The listing builds one solid part. Answer for the finished solid, in the listing's coordinates (mm). Face numbers are marked on the shaded views. A direction names the side the tool comes from. Coordinates: 2 decimals unless noted, no trailing zeros. Order: outer loops, then holes, each group sorted by start corner. A loop starts at its lowest first (then second) coordinate and runs counter-clockwise, first axis right, second up. Notation, with made-up numbers: (2.5, 16) -> (14.5, 16) arc R21 cw to (14.5, 27) -> close; hole circle Ø1 at (14.25, -11). An arc over 180 degrees is marked (long way). Answer in a Markdown table with one row per item.
Autodesk Fusion 360 part; units mm, degrees
sketch "Sketch1" plane through (0, 0, 0) normal (1, 0, 0) x (0, 1, 0)
  line L0 (0, 0) -> (-30, 0)
  line L1 (-30, 0) -> (-30, 15.5)
  line L2 (-30, 15.5) -> (0, 15.5)
  line L3 (0, 15.5) -> (0, 0)
  circle A0 centre (-4, 10.5) radius 1.6
  circle A1 centre (-24, 10.5) radius 1.6
  dimension "d1" = 30
  dimension "d2" = 15.5
  dimension "d3" = 3.2
  dimension "d4" = 3.2
  dimension "d5" = 20
  dimension "d6" = 4
  dimension "d7" = 5
extrude "Extrude1" add sketch "Sketch1" along normal blind 3 makes body 1
sketch "Sketch2" plane through (0, 0, 0) normal (0, 1, 0) x (1, 0, 0)
sketch "Sketch3" plane through (0, -30, 0) normal (0, -1, 0) x (1, 0, 0)
  line L0 (0, 15.5) -> (0, 0)
  line L1 (0, 0) -> (3, 0)
  line L2 (3, 0) -> (3, 15.5)
  line L3 (3, 15.5) -> (0, 15.5)
  line L4 (3, 15.5) -> (15, 15.5)
  line L5 (15, 15.5) -> (15, 0)
  line L6 (15, 0) -> (3, 0)
  line L7 (3, 0) -> (3, 15.5)
  dimension "d10" = 12
extrude "Extrude2" add sketch "Sketch3" against normal blind 3 contours L2 L4 L5 L6 L7 bodies 1
sketch "Sketch4" plane through (15, 0, 0) normal (1, 0, 0) x (0, 1, 0)
  line L0 (-30, 15.5) -> (-30, 0)
  line L1 (-30, 0) -> (-27, 0)
  line L2 (-27, 0) -> (-27, 15.5)
  line L3 (-27, 15.5) -> (-30, 15.5)
  line L4 (-30, 15.5) -> (-43, 15.5)
  line L5 (-43, 15.5) -> (-43, 0)
  line L6 (-43, 0) -> (-30, 0)
  line L7 (-30, 0) -> (-30, 15.5)
  dimension "d13" = 13
extrude "Extrude3" add sketch "Sketch4" along normal blind 3 separate body contours L0 L4 L5 L6 L7 makes body 2
extrude "Extrude4" add 1 faces at (16, -30, 10.3333) along direction (0, 1, 0) blind 3 on bodies 2 bodies 2 1
fillet "Fillet1" radius 1 1 edges at (18, -27, 7.75) on bodies 2
fillet "Fillet2" radius 1 1 edges at (3, -27, 7.75) on bodies 2
fillet "Fillet3" radius 1 1 edges at (1.5, 0, 15.5) on bodies 2
fillet "Fillet4" radius 1 1 edges at (0, -30, 7.75) on bodies 2
fillet "Fillet5" radius 1 1 edges at (15, -30, 7.75) on bodies 2
sketch "Sketch13" plane through (0, -43, 0) normal (0, -1, 0) x (1, 0, 0)
  line L0 (15, 15.5) -> (15, 0)
  line L1 (15, 0) -> (18, 0)
  line L2 (18, 0) -> (18, 15.5)
  line L3 (18, 15.5) -> (15, 15.5)
  line L4 (15, 15.5) -> (46, 15.5)
  line L5 (46, 15.5) -> (46, 0)
  line L6 (46, 0) -> (15, 0)
  line L7 (15, 0) -> (15, 15.5)
  circle A0 centre (43.5, 8) radius 1.6
  circle A1 centre (23.5, 8) radius 1.6
  line L8 (15, 15.5) -> (15, 0)
  line L9 (15, 0) -> (18, 0)
  line L10 (18, 0) -> (18, 15.5)
  line L11 (18, 15.5) -> (15, 15.5)
  dimension "d97" = 31
  dimension "d98" = 15.5
  dimension "d99" = 3.2
  dimension "d101" = 3.2
  dimension "d102" = 20
  dimension "d111" = 7.5
  dimension "d114" = 2.5
extrude "Extrude19" add sketch "Sketch13" along normal blind 3 contours L2 L4 L5 L6 L10 bodies 2
extrude "Extrude20" add 1 faces at (18, -44, 5.1667) along direction (-1, 0, 0) blind 3 on bodies 2 bodies 2
fillet "Fillet8" radius 1 1 edges at (15, -46, 7.75) on bodies 2
fillet "Fillet9" radius 1 1 edges at (18, -43, 7.75) on bodies 2
extrude "Extrude21" add 1 faces at (46, -44, 10.3333) along direction (1, 0, 0) blind 2 on bodies 2 bodies 2
fillet "Fillet11" radius 1 1 edges at (48, -44.5, 15.5) on bodies 2
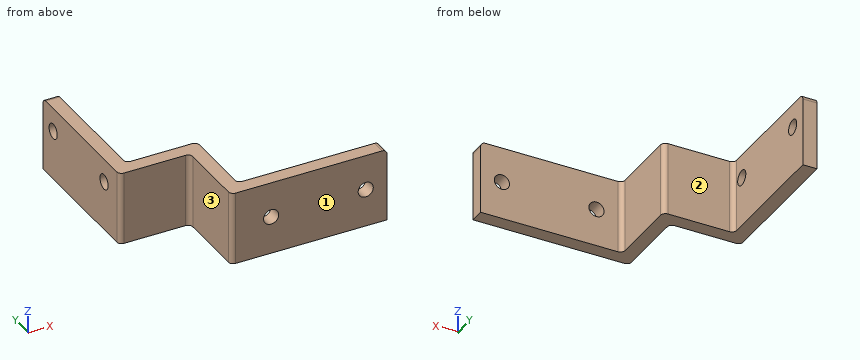
(1) Which of the six approach directions +Z, -Z, +X, -X, +Y, -Y give full straight-line access (tool end or side, diameter ignored) to the marked faces 1, 2 and 3?
Check values:
| item | result |
|---|---|
| face 1 | +Z, -Z, +X, -X, -Y |
| face 2 | +Z, -Z, +X, +Y |
| face 3 | +Z, -Z, -X, -Y |
(2) Find the intervals of material crossed by line 1 along Z through (x, y) = (1.2, -24); line 2 along Z through (x, y) = (43.5, -45.1); line 3 along X through (y, z) = (-39.5, 7), in increasing order. Write a range as from..to.
Check values:
| item | result |
|---|---|
| line 1 | 0..8.9, 12.1..15.5 |
| line 2 | 0..6.4, 9.6..15.5 |
| line 3 | 15..18 |
(3) A cutting plane is placed at C-C, the plane x = 23.5. Determine the outline of the cut face in (y, z).
Check values:
| item | result |
|---|---|
| outline | (-46, 0) -> (-43, 0) -> (-43, 6.4) -> (-46, 6.4) -> close; (-46, 9.6) -> (-43, 9.6) -> (-43, 15.5) -> (-46, 15.5) -> close |
(4) A cutting plane is placed at D-D, the plane y = -13.5. Determine the outline of the cut face in (x, z).
Check values:
| item | result |
|---|---|
| outline | (0, 0) -> (3, 0) -> (3, 15.5) -> (0, 15.5) -> close |
(5) A cutting plane is placed at B-B, the plane z = 10.5. Determine the outline of the cut face in (x, y).
Check values:
| item | result |
|---|---|
| outline | (0, -29) arc R1 ccw to (1, -30) -> (14, -30) arc R1 cw to (15, -31) -> (15, -45) arc R1 ccw to (16, -46) -> (48, -46) -> (48, -43) -> (19, -43) arc R1 cw to (18, -42) -> (18, -28) arc R1 ccw to (17, -27) -> (4, -27) arc R1 cw to (3, -26) -> (3, -25.6) -> (0, -25.6) -> close; (0, -22.4) -> (3, -22.4) -> (3, -5.6) -> (0, -5.6) -> close; (0, -2.4) -> (3, -2.4) -> (3, 0) -> (0, 0) -> close |
(6) A cutting plane is placed at A-A, the plane y = -4. Determine the outline of the cut face in (x, z), then the cut area to 3 significant figures.
Check values:
| item | result |
|---|---|
| outline | (0, 0) -> (3, 0) -> (3, 8.9) -> (0, 8.9) -> close; (0, 12.1) -> (3, 12.1) -> (3, 15.5) -> (0, 15.5) -> close |
| area | 36.9 mm² |
(7) Flat-ended cylindrical pins translate along their axes: pin 1 (3.5 mm diameter, centred on x = 23.5, z = 8, fed in from +Y); pin 2 (3 mm diameter, centred on y = -4, z = 10.5, fed in from +X); pin 3 (4 mm diameter, centred on x = 18, z = 9.5, fed in from +Y); pin 4 (8 mm diameter, centred on y = -12, z = 10.5, fed in from +X). Find the tip coordinate at first contact, or state that the pin passes through.
Check values:
| item | result |
|---|---|
| pin 1 | y = -43 |
| pin 2 | through |
| pin 3 | y = -27 |
| pin 4 | x = 3 |
